Work out the finished part from the listing and answer in its coordinate system (mm). Round coordinates to 2 decimals unless told otherwise and drop trailing zeros. Loops run counter-clockwise (first coordinate to the right, second up) from the corner with the lowest first, then second, coordinate; pieces in that order, holes last. Notation, with made-up numbers: M 62,39 L 97,39 A33 cw 97,71 Z; hole C -14.75,88 d11. An arc over 180 degrees is marked long. One line per item, written item: value.
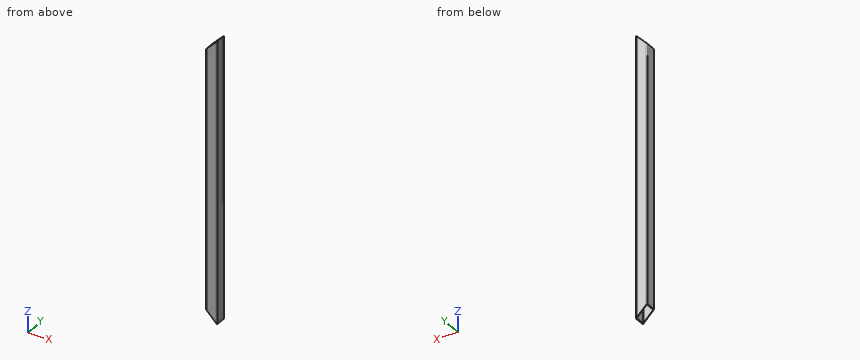
```python
from build123d import *

# Parameters (mm, degrees)
F1_DEPTH      = 500
F3_DEPTH      = 20.001
F3_DEPTH_BACK = 20.001


# Not quite as in the source:
# - a pattern or mirror of a feature is missing from the dataset's text; its kind, count and spacing are read off the source's solid


with BuildPart() as f1:
    # F0 (on Top) → F1 (new body, symmetric)
    with BuildSketch(Plane.XY):
        with BuildLine():
            Line((17, 20), (-17, 20))
            ThreePointArc((-17, 20), (-19.1213203436, 19.1213203436), (-20, 17))
            Line((-20, 17), (-20, -17))
            ThreePointArc((-20, -17), (-19.1213203436, -19.1213203436), (-17, -20))
            Line((-17, -20), (17, -20))
            ThreePointArc((17, -20), (19.1213203436, -19.1213203436), (20, -17))
            Line((20, -17), (20, 17))
            ThreePointArc((20, 17), (19.1213203436, 19.1213203436), (17, 20))
        make_face()
        with BuildLine():
            ThreePointArc((-18, 17), (-17.7071067812, 17.7071067812), (-17, 18))
            Line((-17, 18), (17, 18))
            ThreePointArc((17, 18), (17.7071067812, 17.7071067812), (18, 17))
            Line((18, 17), (18, -17))
            ThreePointArc((18, -17), (17.7071067812, -17.7071067812), (17, -18))
            Line((17, -18), (-17, -18))
            ThreePointArc((-17, -18), (-17.7071067812, -17.7071067812), (-18, -17))
            Line((-18, -17), (-18, 17))
        make_face(mode=Mode.SUBTRACT)
    extrude(amount=F1_DEPTH, both=True)

    # F2 (on Front) → F3 (cut, two sides)
    with BuildSketch(Plane.XZ) as f3_sk:
        Polygon((20, 500), (-20, 500), (-20, 460), align=None)
    f3 = extrude(amount=-F3_DEPTH, mode=Mode.SUBTRACT) + extrude(f3_sk.sketch, amount=F3_DEPTH_BACK, mode=Mode.SUBTRACT)

    # F3_copies: F3 across plane
    add(f3.mirror(Plane(origin=(0, 0, 0), x_dir=(-1, 0, 0), z_dir=(0, 0, -1))), mode=Mode.SUBTRACT)


solid = f1.part
```
1) Find the intervals of material crossed by probe 1 along Y at (x, z) = (16.5, 158.5); probe 2 along X at (y, z) = (17.5, -42), in increasing order. Write a range as from..to.
Check values:
probe 1: -20..-18, 18..20
probe 2: -19.96..-17.87, 17.87..19.96
2) This flat-tipped pin is pushed along its axis until it touches: pin 1 (12 mm diameter, centred on x = 11, y = -7, fed in from -Z). Where does it stop, or does it pass through?
Check values:
pin 1: through
3) Find section A-A (y = 2). Give the vertices of the cut face in (x, z), then the cut area to 3 significant figures.
Check values:
outline: M -20,-460 L -18,-462 L -18,462 L -20,460 Z; M 18,-498 L 20,-500 L 20,500 L 18,498 Z
area: 3,840 mm2
4) Find section C-C (x = -2). Give the vertices of the cut face in (y, z).
Check values:
outline: M -20,-478 L -18,-478 L -18,478 L -20,478 Z; M 18,-478 L 20,-478 L 20,478 L 18,478 Z
5) Find section B-B (z = -367). Give the vertices of the cut face in (x, y), then the cut area to 3 significant figures.
Check values:
outline: M -20,-17 A3 ccw -17,-20 L 17,-20 A3 ccw 20,-17 L 20,17 A3 ccw 17,20 L -17,20 A3 ccw -20,17 Z; hole M -18,-17 A1 ccw -17,-18 L 17,-18 A1 ccw 18,-17 L 18,17 A1 ccw 17,18 L -17,18 A1 ccw -18,17 Z
area: 297 mm2
